The listing builds one solid part. Answer for the finished solid, in the listing's coordinates (mm). Face numbers are marked on the shaded views. A direction names the side the tool comes from. Round coordinates to 2 decimals unless told otherwise and drop trailing zeros. Write each loop counter-clockwise with the first axis right and the second up, starting at its lowest first coordinate (ties: lowest second). Pieces come first, ordered by that corner, then holes. Notation, with made-up numbers: M -7.5,81 L -0.5,81 A23 ccw -0.5,115 Z; hole C -35,-7 d5. An arc over 180 degrees is marked long. One line per item, written item: value. Start each with the question number.
(1) Section D-D (x = 4) is taken. State how many separate pieces and enclosed holes the cut face has, plus the area to 3 significant figures.
(2) Section B-B (x = 9.9) is taken. Determine the outline of the cut face in (y, z).
(3) For the marked faces 1, 2 and 3, determine the directions among +Z, -Z, +X, -X, +Y, -Y from which every point of the face is accessible in a straight line to the end or side of a thin tool.
(4) Section A-A (z = -100) is taken. Determine the outline of the cut face in (x, y).
(5) For a pull along Z with two mould halves and no side action, classify the marked faces 4 and 5 as released by +Z, released by -Z, zero draft, split by the parting line, or undercut.
(6) Given P1, Ø7, axis at x = 10.5, z = -56, coming from the -Y side; P2, Ø5, axis at x = 4, z = -100, coming from the -Y side; P3, Ø1.8, axis at x = 4, z = -22.5, coming from the +Y side; P4, Ø4, axis at x = 5.5, z = -26, coming from the -Y side, each flat-ended and moving along its own axis, determine where each tip first touches the part or whether it passes through.
(7) Section C-C (z = -57) is taken. Determine the outline of the cut face in (x, y), plus the area to 3 significant figures.
(8) Consider probe 1 along Z at (x, y) = (5.75, 2); probe 2 along Y at (x, z) = (4, -4.9); probe 3 along X at (y, z) = (-0.7, -57). Determine where each line is inside the solid, lowest interval first.
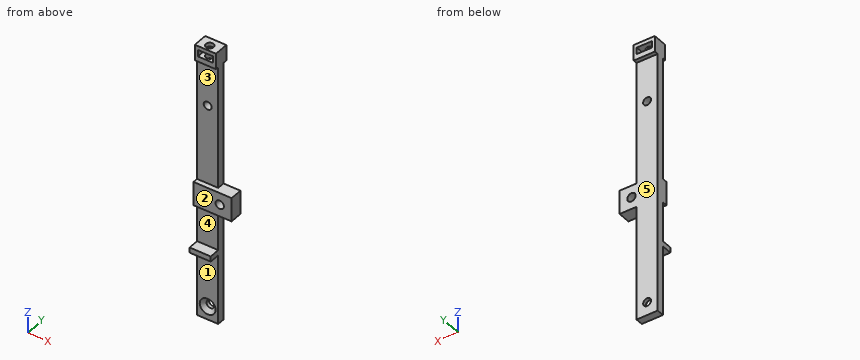
```python
from build123d import *

# Parameters (mm, degrees)
BOSS_EXTRUDE1_DEPTH      = 2.8
CUT_EXTRUDE1_REACH       = 4.8
SKETCH3_R                = 1.5
CHAMFER1_SIZE            = 1.5
SKETCH6_W                = 8
SKETCH6_H                = 6
BOSS_EXTRUDE3_DEPTH      = 1.2
BOSS_EXTRUDE3_DEPTH_BACK = 4.3
SKETCH7_R                = 1.5
CUT_EXTRUDE3_DEPTH       = 6
SKETCH8_W                = 5.7
SKETCH8_H                = 2.5
CUT_EXTRUDE4_DEPTH       = 7
SKETCH9_W                = 14.4
SKETCH9_H                = 9
BOSS_EXTRUDE4_DEPTH      = 4.7
CUT_EXTRUDE5_REACH       = 8.2
SKETCH10_R               = 1.6
SKETCH10_R_2             = 1.5
SKETCH11_W               = 8
SKETCH11_H               = 2
BOSS_EXTRUDE5_DEPTH      = 4


with BuildPart() as part:
    # Sketch2 → Boss-Extrude1 (new body)
    with BuildSketch(Plane(origin=(0, 0, 0), x_dir=(1, 0, 0), z_dir=(0, 1, 0))):
        Polygon((0, 0), (0, 37.522747897), (0, 55), (0, 105), (4, 105), (8, 105), (8, 55), (8, 37.522747897), (8, 0), align=None)
    extrude(amount=BOSS_EXTRUDE1_DEPTH)

    # Sketch3 → Cut-Extrude1 (cut, up to next)
    with BuildSketch(Plane(origin=(0, 2.8, 0), x_dir=(1, 0, 0), z_dir=(0, 1, 0)), mode=Mode.PRIVATE) as cut_extrude1_sk1:
        with Locations(Location((4, 100, 0), (0, 0, 270))):  # turned: the seam where the file's is
            Circle(SKETCH3_R)
    cut_extrude1_tool1 = extrude(cut_extrude1_sk1.sketch, amount=-CUT_EXTRUDE1_REACH, mode=Mode.PRIVATE) & part.part
    add(cut_extrude1_tool1.solids().sort_by_distance((4, 2.8, -100))[0], mode=Mode.SUBTRACT)

    # Chamfer1
    chamfer1_edges = [part.edges().sort_by_distance(p)[0] for p in [
        (4, 0, -101.5),
    ]]
    chamfer(chamfer1_edges, length=CHAMFER1_SIZE)

    # Sketch6 → Boss-Extrude3 (add, two sides)
    with BuildSketch(Plane(origin=(0, 0, 0), x_dir=(-1, 0, 0), z_dir=(0, -1, 0))) as boss_extrude3_sk:
        with Locations((-4, 3)):
            Rectangle(SKETCH6_W, SKETCH6_H)
    extrude(amount=BOSS_EXTRUDE3_DEPTH)
    extrude(boss_extrude3_sk.sketch, amount=-BOSS_EXTRUDE3_DEPTH_BACK)

    # Sketch7 → Cut-Extrude3 (cut)
    with BuildSketch(Plane.XY):
        with Locations((4, 1.1)):
            Circle(SKETCH7_R)
    extrude(amount=-CUT_EXTRUDE3_DEPTH, mode=Mode.SUBTRACT)

    # Sketch8 → Cut-Extrude4 (cut)
    with BuildSketch(Plane(origin=(0, 4.3, 0), x_dir=(1, 0, 0), z_dir=(0, 1, 0))):
        with Locations((4, 2.75)):
            Rectangle(SKETCH8_W, SKETCH8_H)
    extrude(amount=-CUT_EXTRUDE4_DEPTH, mode=Mode.SUBTRACT)

    # Sketch9 → Boss-Extrude4 (add)
    with BuildSketch(Plane(origin=(0, 2.8, 0), x_dir=(1, 0, 0), z_dir=(0, 1, 0))):
        with Locations((7.2, 57)):
            Rectangle(SKETCH9_W, SKETCH9_H)
    extrude(amount=-BOSS_EXTRUDE4_DEPTH)

    # Sketch10 → Cut-Extrude5 (cut, up to next)
    with BuildSketch(Plane.XZ.offset(1.9), mode=Mode.PRIVATE) as cut_extrude5_sk1:
        with Locations(Location((9.9, -57, 0), (0, 0, 270))):  # turned: the seam where the file's is
            Circle(SKETCH10_R)
    cut_extrude5_tool1 = extrude(cut_extrude5_sk1.sketch, amount=-CUT_EXTRUDE5_REACH, mode=Mode.PRIVATE) & part.part
    add(cut_extrude5_tool1.solids().sort_by_distance((9.9, -1.9, -57))[0], mode=Mode.SUBTRACT)
    # Sketch10 → Cut-Extrude5 (cut, up to next)
    with BuildSketch(Plane.XZ.offset(1.9), mode=Mode.PRIVATE) as cut_extrude5_sk2:
        with Locations(Location((4, -22.5, 0), (0, 0, 270))):  # turned: the seam where the file's is
            Circle(SKETCH10_R_2)
    cut_extrude5_tool2 = extrude(cut_extrude5_sk2.sketch, amount=-CUT_EXTRUDE5_REACH, mode=Mode.PRIVATE) & part.part
    add(cut_extrude5_tool2.solids().sort_by_distance((4, -1.9, -22.5))[0], mode=Mode.SUBTRACT)

    # Sketch11 → Boss-Extrude5 (add)
    with BuildSketch(Plane.XZ):
        with Locations((4, -77.5)):
            Rectangle(SKETCH11_W, SKETCH11_H)
    extrude(amount=BOSS_EXTRUDE5_DEPTH)


solid = part.part
```
Recorded:
1. separate pieces: 6
1. enclosed holes: 0
1. area: 292 mm2
2. outline: M -1.9,-61.5 L 2.8,-61.5 L 2.8,-58.6 L -1.9,-58.6 Z; M -1.9,-55.4 L 2.8,-55.4 L 2.8,-52.5 L -1.9,-52.5 Z
3. face 1: -Z, +X, -X, -Y
3. face 2: +Z, +X, -X, -Y
3. face 3: +X, -X, -Y
4. outline: M 0,0 L 1,0 L 2.5,1.5 L 2.5,2.8 L 0,2.8 Z; M 5.5,1.5 L 7,0 L 8,0 L 8,2.8 L 5.5,2.8 Z
5. face 4: undercut
5. face 5: zero draft
6. P1: stops at y = -1.9
6. P2: stops at y = 0.5
6. P3: passes through
6. P4: stops at y = 0
7. outline: M 0,-1.9 L 8.3,-1.9 L 8.3,2.8 L 0,2.8 Z; M 11.5,-1.9 L 14.4,-1.9 L 14.4,2.8 L 11.5,2.8 Z
7. area: 52.6 mm2
8. probe 1: z = -105 to -4, -1.5 to 0
8. probe 2: y = -1.2 to -0.4, 2.6 to 4.3
8. probe 3: x = 0 to 8.3, 11.5 to 14.4
